Verification items for the finished model (mm, model axes). A direction names the side the tool comes from. Coordinates: 2 decimals unless noted, no trailing zeros. Write each loop counter-clockwise with the first axis right and the second up, starting at its lowest first coordinate (ties: lowest second). Pieces come first, ordered by that corner, then holes. Notation, with made-up numbers: (81.25, 37.5) -> (135.25, 37.5) arc R24 ccw to (135.25, 54.5) -> close; hole circle Ø7 at (-9.75, 85). An arc over 180 degrees is marked (long way). Answer in a Markdown table with one row per item.
```python
from build123d import *

# Parameters (mm, degrees)
SKETCH2_W           = 177.8
SKETCH2_H           = 101.6
BOSS_EXTRUDE1_DEPTH = 5
SKETCH3_W           = 177.8
SKETCH3_H           = 5
BOSS_EXTRUDE3_DEPTH = 25.4
SKETCH4_R           = 5
CUT_EXTRUDE1_DEPTH  = 208.025505675
FILLET1_R           = 12.7


with BuildPart() as part:
    # Sketch2 → Boss-Extrude1 (new body)
    with BuildSketch(Plane(origin=(0, 0, 0), x_dir=(1, 0, 0), z_dir=(0, 1, 0))):
        with Locations((88.9, 50.8)):
            Rectangle(SKETCH2_W, SKETCH2_H)
    extrude(amount=BOSS_EXTRUDE1_DEPTH)

    # Sketch3 → Boss-Extrude3 (add)
    with BuildSketch(Plane(origin=(0, 5, 0), x_dir=(1, 0, 0), z_dir=(0, 1, 0))):
        with Locations((88.9, 2.5)):
            Rectangle(SKETCH3_W, SKETCH3_H)
        with Locations((88.9, 99.1)):
            Rectangle(SKETCH3_W, SKETCH3_H)
    extrude(amount=BOSS_EXTRUDE3_DEPTH)

    # Sketch4 → Cut-Extrude1 (cut, through all)
    with BuildSketch(Plane.XY):
        with Locations((12.7, 17.7)):
            Circle(SKETCH4_R)
        with BuildLine():
            Line((50.8, 22.7), (152.4, 22.7))
            ThreePointArc((152.4, 22.7), (157.4, 17.7), (152.4, 12.7))
            Line((152.4, 12.7), (50.8, 12.7))
            ThreePointArc((50.8, 12.7), (45.8, 17.7), (50.8, 22.7))
        make_face()
    extrude(amount=-CUT_EXTRUDE1_DEPTH, mode=Mode.SUBTRACT)

    # Fillet1
    fillet1_edges = [part.edges().sort_by_distance(p)[0] for p in [
        (0, 30.4, -2.5),
        (177.8, 30.4, -2.5),
        (0, 30.4, -99.1),
        (177.8, 30.4, -99.1),
    ]]
    fillet(fillet1_edges, radius=FILLET1_R)


solid = part.part
```
1. Section check B-B, the plane y = 10. Record the boundary of the cut face in (x, z), plus the area to 3 significant figures.
Geometry says:
| item | result |
|---|---|
| outline | (0, -101.6) -> (177.8, -101.6) -> (177.8, -96.6) -> (0, -96.6) -> close; (0, -5) -> (177.8, -5) -> (177.8, 0) -> (0, 0) -> close |
| area | 1,780 mm^2 |
2. Section check C-C, the plane y = 21. Record the boundary of the cut face in (x, z).
Geometry says:
| item | result |
|---|---|
| outline | (0.44, -101.6) -> (8.94, -101.6) -> (8.94, -96.6) -> (0.44, -96.6) -> close; (0.44, -5) -> (8.94, -5) -> (8.94, 0) -> (0.44, 0) -> close; (16.46, -101.6) -> (47.04, -101.6) -> (47.04, -96.6) -> (16.46, -96.6) -> close; (16.46, -5) -> (47.04, -5) -> (47.04, 0) -> (16.46, 0) -> close; (156.16, -101.6) -> (177.36, -101.6) -> (177.36, -96.6) -> (156.16, -96.6) -> close; (156.16, -5) -> (177.36, -5) -> (177.36, 0) -> (156.16, 0) -> close |
3. Tool access check on faces 5 (the flat face through (0, 4.8, -38.8)), 6 (the flat face through (88, 5, -51)), 7 (the flat face through (102, 12.7, -2)). Record the directions out of +Z, -Z, +X, -X, +Y, -Y that give a thin tool (end or side, any length) a straight path to the whole face; none if there is none.
Geometry says:
| item | result |
|---|---|
| face 5 | +Z, -Z, -X, +Y, -Y |
| face 6 | +X, -X, +Y |
| face 7 | +Z, -Z |
4. Mould release check, pull along X, two halves, no side actions. Record for faces 1 (the cylindrical face through (173.98, 26.78, -99.14)), 2 (the flat face through (88, 30.4, -3)), 3 (the flat face through (101, 22.7, -99)), 4 (the cylindrical face through (7.705, 17.92, -2.465)): released by +X, released by -X, zero draft, split by the parting line, or undercut.
Geometry says:
| item | result |
|---|---|
| face 1 | released by +X |
| face 2 | zero draft |
| face 3 | undercut |
| face 4 | undercut |
5. Section check A-A, the plane x = 139. Record the boundary of the cut face in (y, z), plus the area to 3 significant figures.
Geometry says:
| item | result |
|---|---|
| outline | (0, -101.6) -> (12.7, -101.6) -> (12.7, -96.6) -> (5, -96.6) -> (5, -5) -> (12.7, -5) -> (12.7, 0) -> (0, 0) -> close; (22.7, -101.6) -> (30.4, -101.6) -> (30.4, -96.6) -> (22.7, -96.6) -> close; (22.7, -5) -> (30.4, -5) -> (30.4, 0) -> (22.7, 0) -> close |
| area | 662 mm^2 |
6. Thickness scan on line 1 (Z direction, x = 115, y = 9); line 2 (X direction, y = 17, z = -3); line 3 (Y direction, x = 12.7, z = -3.55). Record the ranges inside material, lowest first. Write a range as from..to.
Geometry says:
| item | result |
|---|---|
| line 1 | -101.6..-96.6, -5..0 |
| line 2 | 0..7.75, 17.65..45.85, 157.35..177.8 |
| line 3 | 0..12.7, 22.7..30.4 |
7. Section check D-D, the plane z = -70. Record the boundary of the cut face in (x, y), plus the area to 3 significant figures.
Geometry says:
| item | result |
|---|---|
| outline | (0, 0) -> (177.8, 0) -> (177.8, 5) -> (0, 5) -> close |
| area | 889 mm^2 |
8. Depth check by flat-ended pin: P1, Ø5, axis at x = 20, z = -34.5, coming from the +Y side. Enter the tip coordinate at first touch or a pass-through.
Geometry says:
| item | result |
|---|---|
| P1 | y = 5 |
